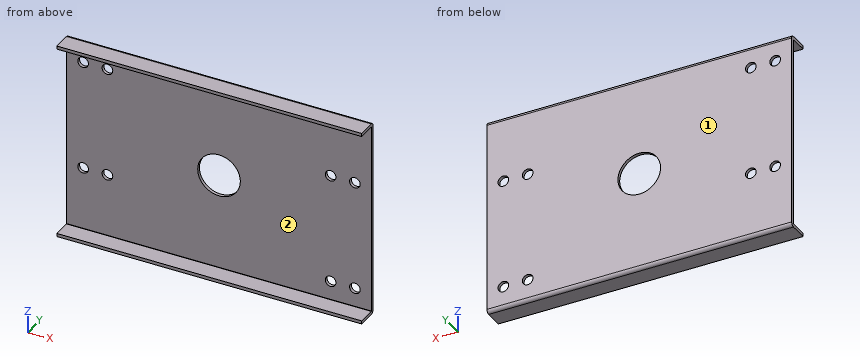
from build123d import *

# Parameters (mm, degrees)
SKETCH2_W                      = 143
SKETCH2_H                      = 93
BASE_FLANGE1_DEPTH             = 1.5
EDGE_FLANGE1_STRIP_W           = 6.2
EDGE_FLANGE1_STRIP_H           = 1.5
EDGE_FLANGE1_STRIP_CUT_DEPTH   = 143
EDGE_FLANGE1_STRIP_2_W         = 6.2
EDGE_FLANGE1_STRIP_2_H         = 1.5
EDGE_FLANGE1_STRIP_CUT_2_DEPTH = 143
EDGE_FLANGE1_DEPTH             = 143
EDGE_FLANGE1_BEND_DEPTH        = 143
SKETCH13_R                     = 10
CUT_EXTRUDE1_DEPTH             = 1.5
SKETCH14_R                     = 2.5
CUT_EXTRUDE2_DEPTH             = 1.5


# Sheet-metal steps are written as plain solids
with BuildPart() as part:
    # Sketch2 → Base-Flange1 (new body)
    with BuildSketch(Plane(origin=(0, 0, 0), x_dir=(1, 0, 0), z_dir=(0, 1, 0))):
        Rectangle(SKETCH2_W, SKETCH2_H)
    extrude(amount=-BASE_FLANGE1_DEPTH)

    # Edge-Flange1 strip (across the edge) → Edge-Flange1 strip cut (cut)
    with BuildSketch(Plane(origin=(71.5, -1.5, 46.5), x_dir=(0, 0, -1), z_dir=(-1, 0, 0))):
        with Locations((-1.5, -0.75)):
            Rectangle(EDGE_FLANGE1_STRIP_W, EDGE_FLANGE1_STRIP_H)
    extrude(amount=EDGE_FLANGE1_STRIP_CUT_DEPTH, mode=Mode.SUBTRACT)

    # Edge-Flange1 strip 2 (across the edge) → Edge-Flange1 strip cut 2 (cut)
    with BuildSketch(Plane(origin=(-71.5, -1.5, -46.5), x_dir=(0, 0, 1), z_dir=(1, 0, 0))):
        with Locations((-1.5, -0.75)):
            Rectangle(EDGE_FLANGE1_STRIP_2_W, EDGE_FLANGE1_STRIP_2_H)
    extrude(amount=EDGE_FLANGE1_STRIP_CUT_2_DEPTH, mode=Mode.SUBTRACT)

    # Edge-Flange1 section (across the edge) → Edge-Flange1 (add)
    with BuildSketch(Plane(origin=(71.5, -1.5, 46.5), x_dir=(0, 0, -1), z_dir=(-1, 0, 0))):
        with BuildLine():
            Line((0, 0.1), (0, 8.5))
            Line((0, 8.5), (1.5, 8.5))
            Line((1.5, 8.5), (1.5, 0.1))
            ThreePointArc((1.5, 0.1), (1.529289322, 0.029289322), (1.6, 0))
            Line((1.6, 0), (1.6, -1.5))
            ThreePointArc((1.6, -1.5), (0.46862915, -1.03137085), (0, 0.1))
        make_face()
    extrude(amount=EDGE_FLANGE1_DEPTH)

    # Edge-Flange1 section 2 (across the edge) → Edge-Flange1 bend (add)
    with BuildSketch(Plane(origin=(-71.5, -1.5, -46.5), x_dir=(0, 0, 1), z_dir=(1, 0, 0))):
        with BuildLine():
            Line((0, 0.1), (0, 8.5))
            Line((0, 8.5), (1.5, 8.5))
            Line((1.5, 8.5), (1.5, 0.1))
            ThreePointArc((1.5, 0.1), (1.529289322, 0.029289322), (1.6, 0))
            Line((1.6, 0), (1.6, -1.5))
            ThreePointArc((1.6, -1.5), (0.46862915, -1.03137085), (0, 0.1))
        make_face()
    extrude(amount=EDGE_FLANGE1_BEND_DEPTH)

    # Sketch13 → Cut-Extrude1 (cut)
    with BuildSketch(Plane(origin=(0, 0, 0), x_dir=(1, 0, 0), z_dir=(0, 1, 0))):
        with Locations(Location((0, 0, 0), (0, 0, 270))):
            Circle(SKETCH13_R)
    extrude(amount=-CUT_EXTRUDE1_DEPTH, mode=Mode.SUBTRACT)

    # Sketch14 → Cut-Extrude2 (cut)
    with BuildSketch(Plane(origin=(0, 0, 0), x_dir=(1, 0, 0), z_dir=(0, 1, 0))):
        with Locations(Location((63.775, 36.1, 0), (0, 0, 270))):
            Circle(SKETCH14_R)
        with Locations(Location((52.365, 36.1, 0), (0, 0, 270))):
            Circle(SKETCH14_R)
        with Locations(Location((52.365, -15.41, 0), (0, 0, 270))):
            Circle(SKETCH14_R)
        with Locations(Location((63.775, -15.41, 0), (0, 0, 270))):
            Circle(SKETCH14_R)
        with Locations(Location((-63.775, -36.1, 0), (0, 0, 270))):
            Circle(SKETCH14_R)
        with Locations(Location((-52.365, -36.1, 0), (0, 0, 270))):
            Circle(SKETCH14_R)
        with Locations(Location((-52.365, 15.41, 0), (0, 0, 270))):
            Circle(SKETCH14_R)
        with Locations(Location((-63.775, 15.41, 0), (0, 0, 270))):
            Circle(SKETCH14_R)
    extrude(amount=-CUT_EXTRUDE2_DEPTH, mode=Mode.SUBTRACT)


solid = part.part
For this review, take the finished solid that the model builds, in its own axes (mm). Face numbers are marked on the shaded views. Round coordinates to 2 decimals unless told otherwise and drop trailing zeros. Write each loop counter-clockwise with the first axis right and the second up, starting at its lowest first coordinate (ties: lowest second). Pieces come first, ordered by that corner, then holes. Notation, with made-up numbers: (-17, 85.25) - (41, 85.25) arc R22 ccw to (41, 91.25) - close; hole circle Ø4 at (63.25, 18.5). An arc over 180 degrees is marked (long way). Use a Markdown table: item, result.
Q1. Clearance check with flat-ended pins moving along their axes: pin 1 (8 mm diameter, centred on x = 63.775, z = -36.1, fed in from +Y); pin 2 (6.5 mm diameter, centred on x = -52.365, z = -15.41, fed in from -Y). State where each tip first meets the part, or that it passes through.
Derived:
| item | result |
|---|---|
| pin 1 | stops at y = 0 |
| pin 2 | stops at y = -1.5 |
Q2. The part is to be moulded in two halves that separate along Z. For the marked faces 1 and 2, say which applies: pulls with the +Z half, pulls with the -Z half, needs draft (parallel to the pull), parting line crosses it, or undercut.
Derived:
| item | result |
|---|---|
| face 1 | needs draft |
| face 2 | undercut |
Q3. We need section B-B (x = 0). Give the boundary of the cut face in (y, z), plus the area to 3 significant figures.
Derived:
| item | result |
|---|---|
| outline | (-10, -46.5) - (-1.6, -46.5) arc R1.6 ccw to (0, -44.9) - (0, -10) - (-1.5, -10) - (-1.5, -44.9) arc R0.1 cw to (-1.6, -45) - (-10, -45) - close; (-10, 45) - (-1.6, 45) arc R0.1 cw to (-1.5, 44.9) - (-1.5, 10) - (0, 10) - (0, 44.9) arc R1.6 ccw to (-1.6, 46.5) - (-10, 46.5) - close |
| area | 134 mm2 |
Q4. We need section A-A (z = 0). Give the boundary of the cut face in (x, y).
Derived:
| item | result |
|---|---|
| outline | (-71.5, -1.5) - (-10, -1.5) - (-10, 0) - (-71.5, 0) - close; (10, -1.5) - (71.5, -1.5) - (71.5, 0) - (10, 0) - close |
Q5. We need section D-D (z = -36.1). Give the boundary of the cut face in (x, y) (3 decimals).
Derived:
| item | result |
|---|---|
| outline | (-71.5, -1.5) - (49.865, -1.5) - (49.865, 0) - (-71.5, 0) - close; (54.865, -1.5) - (61.275, -1.5) - (61.275, 0) - (54.865, 0) - close; (66.275, -1.5) - (71.5, -1.5) - (71.5, 0) - (66.275, 0) - close |
Q6. Wall thickness on line 1 along X through (y, z) = (-0.4, -36.1) (3 decimals); line 2 along X through (y, z) = (-0.35, 36.1) (3 decimals); line 3 along Z through (x, y) = (12, -5): over which ranges is each line inside the solid? List them lowest first.
Derived:
| item | result |
|---|---|
| line 1 | x = -71.5 to 49.865, 54.865 to 61.275, 66.275 to 71.5 |
| line 2 | x = -71.5 to -66.275, -61.275 to -54.865, -49.865 to 71.5 |
| line 3 | z = -46.5 to -45, 45 to 46.5 |
Q7. We need section C-C (y = -3.25). Give the boundary of the cut face in (x, z).
Derived:
| item | result |
|---|---|
| outline | (-71.5, -46.5) - (71.5, -46.5) - (71.5, -45) - (-71.5, -45) - close; (-71.5, 45) - (71.5, 45) - (71.5, 46.5) - (-71.5, 46.5) - close |
